Can you work these out from the drawing? Everything is in mm from the part's minimum corner. A direction names the side the tool comes from. Round coordinates to 2 decimals unless told otherwise and drop trailing zeros. Order: outer loops, then holes, each group sorted by start corner. A loop starts at its lowest first (then second) coordinate and runs counter-clockwise, first axis right, second up. Notation, with made-up numbers: (59, 15) - (87, 15) arc R21 ccw to (87, 29) - close; hole circle Ø9 at (40, 41.5). An arc over 180 degrees is marked (long way). Answer as a JSON object with one key per item and string values.
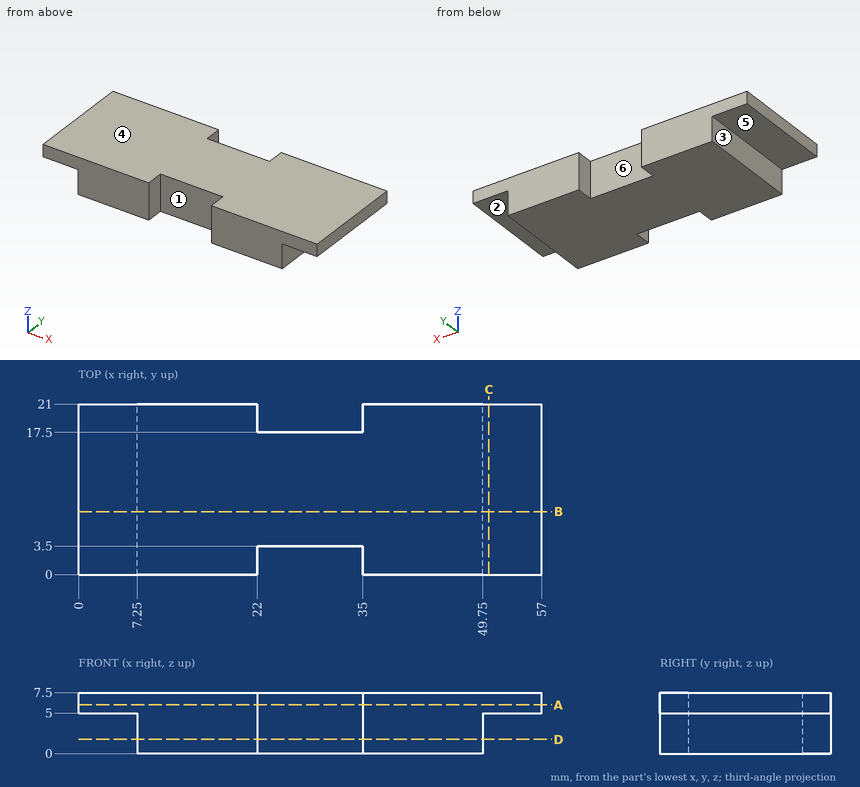
1. For the marked faces 4, 5 and 6, which set-ups out of +Z, -Z, +X, -X, +Y, -Y let a thin tool reach every point of the face, with its end or its side?
Responses:
{"face 4": "+Z, +X, -X, +Y, -Y", "face 5": "-Z, -X, +Y, -Y", "face 6": "+Z, -Z, +Y"}
2. Imagine slicing it at D-D (z = 1.75). List the corners of the cut face in (x, y) for me, plus the area to 4 significant figures.
Responses:
{"outline": "(7.25, 0) - (22, 0) - (22, 3.5) - (35, 3.5) - (35, 0) - (49.75, 0) - (49.75, 21) - (35, 21) - (35, 17.5) - (22, 17.5) - (22, 21) - (7.25, 21) - close", "area": "801.5 mm2"}
3. Thinking about a two-plate mould opening in X: for the marked faces 1, 2 and 3, which applies, pulls with the +X half, pulls with the -X half, needs draft (parallel to the pull), parting line crosses it, or undercut?
Responses:
{"face 1": "undercut", "face 2": "needs draft", "face 3": "pulls with the -X half"}
4. Imagine slicing it at C-C (x = 50.5). List the corners of the cut face in (y, z) for me.
Responses:
{"outline": "(0, 5) - (21, 5) - (21, 7.5) - (0, 7.5) - close"}
5. Imagine slicing it at B-B (y = 7.75). List the corners of the cut face in (x, z) for me, plus the area to 3 significant figures.
Responses:
{"outline": "(0, 5) - (7.25, 5) - (7.25, 0) - (49.75, 0) - (49.75, 5) - (57, 5) - (57, 7.5) - (0, 7.5) - close", "area": "355 mm2"}
6. For P1, Ø1.8, axis at y = 1, z = 4, coming from the +X side; P2, Ø2.5, axis at y = 13.5, z = 2.5, coming from the -X side; P3, Ø8, axis at x = 54, y = 10.5, coming from the -Z side, each with a flat end and sliding along its axis, tell me the tip position at first contact or that it passes through.
Responses:
{"P1": "x = 49.75", "P2": "x = 7.25", "P3": "z = 5"}
7. If I drill on L1, parallel to Z at x = 52, y = 16.5; L2, parallel to X at y = 1, z = 2.75; L3, parallel to X at y = 19, z = 5.25, over which ranges is the centre line in solid material (lowest first)? Write a range as [from, to].
Responses:
{"L1": "[5, 7.5]", "L2": "[7.25, 22], [35, 49.75]", "L3": "[0, 22], [35, 57]"}
8. Imagine slicing it at A-A (z = 6). List the corners of the cut face in (x, y) for me, plus the area to 3 significant figures.
Responses:
{"outline": "(0, 0) - (22, 0) - (22, 3.5) - (35, 3.5) - (35, 0) - (57, 0) - (57, 21) - (35, 21) - (35, 17.5) - (22, 17.5) - (22, 21) - (0, 21) - close", "area": "1,110 mm2"}
